from build123d import *

# Parameters (mm, degrees)
SKETCH2_R           = 2.5
BOSS_EXTRUDE1_DEPTH = 150


with BuildPart() as part:
    # Sketch2 → Boss-Extrude1 (new body)
    with BuildSketch(Plane.XY):
        with BuildLine():
            Line((-10, -10), (-3.1, -10))
            Line((-3.1, -10), (-3.1, -7.81857447))
            Line((-3.1, -7.81857447), (-4.285374034, -7.81857447))
            ThreePointArc((-4.285374034, -7.81857447), (-5.210402021, -7.198473435), (-4.988208383, -6.107220917))
            Line((-4.988208383, -6.107220917), (-2.819718275, -3.96470075))
            Line((-2.819718275, -3.96470075), (0, -3.96470075))
            Line((0, -3.96470075), (2.782738033, -3.96470075))
            Line((2.782738033, -3.96470075), (5.105242131, -6.103332486))
            ThreePointArc((5.105242131, -6.103332486), (5.359419929, -7.202533996), (4.427854938, -7.838959152))
            Line((4.427854938, -7.838959152), (3.1, -7.838959152))
            Line((3.1, -7.838959152), (3.1, -10))
            Line((3.1, -10), (10, -10))
            Line((10, -10), (10, -3.1))
            Line((10, -3.1), (7.81857447, -3.1))
            Line((7.81857447, -3.1), (7.81857447, -4.285374034))
            ThreePointArc((7.81857447, -4.285374034), (7.198473435, -5.210402021), (6.107220917, -4.988208383))
            Line((6.107220917, -4.988208383), (3.96470075, -2.819718275))
            Line((3.96470075, -2.819718275), (3.96470075, 0))
            Line((3.96470075, 0), (3.96470075, 2.782738033))
            Line((3.96470075, 2.782738033), (6.103332486, 5.105242131))
            ThreePointArc((6.103332486, 5.105242131), (7.202533996, 5.359419929), (7.838959152, 4.427854938))
            Line((7.838959152, 4.427854938), (7.838959152, 3.1))
            Line((7.838959152, 3.1), (10, 3.1))
            Line((10, 3.1), (10, 10))
            Line((10, 10), (3.1, 10))
            Line((3.1, 10), (3.1, 7.81857447))
            Line((3.1, 7.81857447), (4.285374034, 7.81857447))
            ThreePointArc((4.285374034, 7.81857447), (5.210402021, 7.198473435), (4.988208383, 6.107220917))
            Line((4.988208383, 6.107220917), (2.819718275, 3.96470075))
            Line((2.819718275, 3.96470075), (0, 3.96470075))
            Line((0, 3.96470075), (-2.782738033, 3.96470075))
            Line((-2.782738033, 3.96470075), (-5.105242131, 6.103332486))
            ThreePointArc((-5.105242131, 6.103332486), (-5.359419929, 7.202533996), (-4.427854938, 7.838959152))
            Line((-4.427854938, 7.838959152), (-3.1, 7.838959152))
            Line((-3.1, 7.838959152), (-3.1, 10))
            Line((-3.1, 10), (-10, 10))
            Line((-10, 10), (-10, 3.1))
            Line((-10, 3.1), (-7.81857447, 3.1))
            Line((-7.81857447, 3.1), (-7.81857447, 4.285374034))
            ThreePointArc((-7.81857447, 4.285374034), (-7.198473435, 5.210402021), (-6.107220917, 4.988208383))
            Line((-6.107220917, 4.988208383), (-3.96470075, 2.819718275))
            Line((-3.96470075, 2.819718275), (-3.96470075, 0))
            Line((-3.96470075, 0), (-3.96470075, -2.782738033))
            Line((-3.96470075, -2.782738033), (-6.103332486, -5.105242131))
            ThreePointArc((-6.103332486, -5.105242131), (-7.202533996, -5.359419929), (-7.838959152, -4.427854938))
            Line((-7.838959152, -4.427854938), (-7.838959152, -3.1))
            Line((-7.838959152, -3.1), (-10, -3.1))
            Line((-10, -3.1), (-10, -10))
        make_face()
        Circle(SKETCH2_R, mode=Mode.SUBTRACT)
    extrude(amount=BOSS_EXTRUDE1_DEPTH)


solid = part.part
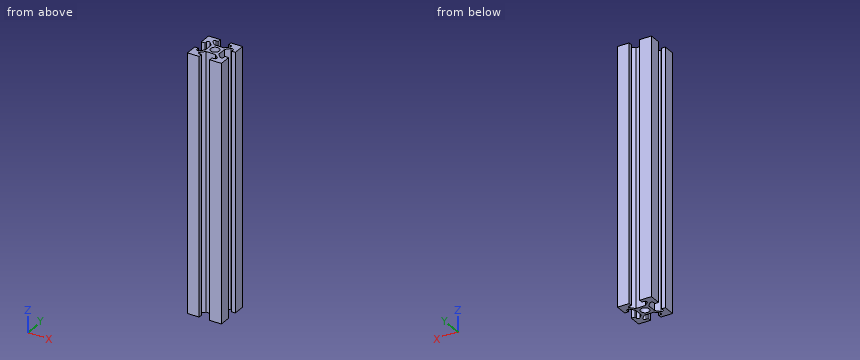
Geometry: final body of the model. Coordinates: model frame, mm. Round coordinates to 2 decimals unless told otherwise and drop trailing zeros. Write each loop counter-clockwise with the first axis right and the second up, starting at its lowest first coordinate (ties: lowest second). Pieces come first, ordered by that corner, then holes. Notation, with made-up numbers: M 75.25,-32 L 95.25,-32 A16 cw 95.25,-26 Z; hole C 0.25,21.25 d4. An arc over 180 degrees is marked long. Write item = value, one per line.
Item 1: Section query A-A on y = 0. Return loops of the section in (x, z), then the cut area to 3 significant figures.
Findings:
outline = M -3.96,0 L -2.5,0 L -2.5,150 L -3.96,150 Z; M 2.5,0 L 3.96,0 L 3.96,150 L 2.5,150 Z
area = 439 mm^2
Item 2: Pin query (flat end, axial travel): P1, Ø3, axis at y = 1, z = 92, coming from the -X side; P2, Ø3, axis at x = 0, z = 80, coming from the +Y side; P3, Ø3, axis at y = -0.5, z = 28.5, coming from the +X side. Return the tip coordinate at first contact, or that it passes through.
Findings:
P1 = -3.96
P2 = 3.96
P3 = 3.96
Item 3: Material intervals for line 1 along Y through (x, z) = (0, 82); line 2 along Y through (x, z) = (-8.25, 20); line 3 along X through (y, z) = (-5, 140.5), sorted ascending. Write a range as [from, to].
Findings:
line_1 = [-3.96, -2.5], [2.5, 3.96]
line_2 = [-10, -3.1], [3.1, 10]
line_3 = [-10, -7.66], [-6.01, -3.87], [3.91, 6.12], [7.52, 10]
